```python
from build123d import *

# Parameters (mm, degrees)
IZIM1_W                     = 100
IZIM1_H                     = 120
Y_KSEKLIK_EKSTR_ZYON1_DEPTH = 20
Y_KSEKLIK_EKSTR_ZYON2_DEPTH = 120
Y_KSEKLIK_EKSTR_ZYON3_DEPTH = 20
RADYUS1_R                   = 10
RADYUS2_R                   = 15
IZIM3_R                     = 20
Y_KSEKLIK_EKSTR_ZYON4_DEPTH = 30
IZIM4_R                     = 5
Y_KSEKLIK_EKSTR_ZYON5_DEPTH = 10
Y_KSEKLIK_EKSTR_ZYON6_START = 30
IZIM5_R                     = 20
Y_KSEKLIK_EKSTR_ZYON6_DEPTH = 30
Y_KSEKLIK_EKSTR_ZYON7_START = 10
IZIM6_R                     = 5
Y_KSEKLIK_EKSTR_ZYON7_DEPTH = 10


with BuildPart() as part:
    # Çizim1 → Yükseklik-Ekstrüzyon1 (new body)
    with BuildSketch(Plane.XY):
        Rectangle(IZIM1_W, IZIM1_H)
    extrude(amount=Y_KSEKLIK_EKSTR_ZYON1_DEPTH)

    # Çizim1<3> → Yükseklik-Ekstrüzyon2 (add)
    with BuildSketch(Plane.XY):
        with BuildLine():
            Line((-50, -60), (-50, 60))
            ThreePointArc((-50, 60), (-110, 0), (-50, -60))
        make_face()
    extrude(amount=Y_KSEKLIK_EKSTR_ZYON2_DEPTH)

    # Çizim2 → Yükseklik-Ekstrüzyon3 (add)
    with BuildSketch(Plane.XY.offset(120)):
        with BuildLine():
            Line((-50, -60), (50, -60))
            Line((50, -60), (50, 60))
            Line((50, 60), (-50, 60))
            ThreePointArc((-50, 60), (-110, 0), (-50, -60))
        make_face()
    extrude(amount=Y_KSEKLIK_EKSTR_ZYON3_DEPTH)

    # Radyus1
    radyus1_edges = [part.edges().sort_by_distance(p)[0] for p in [
        (-50, 0, 120),
        (-50, 0, 20),
    ]]
    fillet(radyus1_edges, radius=RADYUS1_R)

    # Radyus2
    radyus2_edges = [part.edges().sort_by_distance(p)[0] for p in [
        (50, -60, 130),
        (50, 60, 130),
        (50, 60, 10),
        (50, -60, 10),
    ]]
    fillet(radyus2_edges, radius=RADYUS2_R)

    # Çizim3 → Yükseklik-Ekstrüzyon4 (add)
    with BuildSketch(Plane.XY.offset(20)):
        Circle(IZIM3_R)
    extrude(amount=Y_KSEKLIK_EKSTR_ZYON4_DEPTH)

    # Çizim4 → Yükseklik-Ekstrüzyon5 (add)
    with BuildSketch(Plane.XY.offset(50)):
        Circle(IZIM4_R)
    extrude(amount=Y_KSEKLIK_EKSTR_ZYON5_DEPTH)

    # Çizim5 → Yükseklik-Ekstrüzyon6 (add)
    with BuildSketch(Plane(origin=(0, 0, 120), x_dir=(1, 0, 0), z_dir=(0, 0, -1)).offset(Y_KSEKLIK_EKSTR_ZYON6_START)):
        Circle(IZIM5_R)
    extrude(amount=-Y_KSEKLIK_EKSTR_ZYON6_DEPTH)

    # Çizim6 → Yükseklik-Ekstrüzyon7 (add)
    with BuildSketch(Plane(origin=(0, 0, 90), x_dir=(1, 0, 0), z_dir=(0, 0, -1)).offset(Y_KSEKLIK_EKSTR_ZYON7_START)):
        Circle(IZIM6_R)
    extrude(amount=-Y_KSEKLIK_EKSTR_ZYON7_DEPTH)


solid = part.part
```
Check sheet for the modelled part. Datum: model origin and axes. Units: mm. A direction names the side the tool comes from. Coordinates: 2 decimals unless noted, no trailing zeros. Write each loop counter-clockwise with the first axis right and the second up, starting at its lowest first coordinate (ties: lowest second). Pieces come first, ordered by that corner, then holes. Notation, with made-up numbers: (11, 43) -> (62, 43) arc R16 cw to (62, 54) -> close; hole circle Ø9 at (47, 44.25). An arc over 180 degrees is marked (long way). Use a Markdown table: item, result.
1. Scan lines: line 1 along Z through (x, y) = (-18.5, 17); line 2 along X through (y, z) = (0.5, 59.5); line 3 along Z through (x, y) = (-12, 4). Record each from-to range of solid material in increasing order.
Reported:
| item | result |
|---|---|
| line 1 | z = 0 to 20, 120 to 140 |
| line 2 | x = -110 to -50, -4.97 to 4.97 |
| line 3 | z = 0 to 50, 90 to 140 |
2. Tool access check on faces 3 (the cylindrical face through (45.72, -55.49, 10.14)), 4 (the flat face through (4, 4, 90)), 5 (the flat face through (-50, -1, 69)), 6 (the flat face through (50, -1, 10)), 7 (the flat face through (0, 0, 60)). Record the directions out of +Z, -Z, +X, -X, +Y, -Y that give a thin tool (end or side, any length) a straight path to the whole face; none if there is none.
Reported:
| item | result |
|---|---|
| face 3 | +Z, -Z, +X, -Y |
| face 4 | none |
| face 5 | +Y, -Y |
| face 6 | +Z, -Z, +X, +Y, -Y |
| face 7 | +X, +Y, -Y |
3. Go/stop test with flat-tipped pins: pin 1 Ø10 at (x, z) = (-13, 78) entering from -Y; pin 2 Ø5 at (y, z) = (36, 23) entering from -X; pin 3 Ø8 at (y, z) = (32.5, 87) entering from +X. Record where each tip stops, or that it passes through.
Reported:
| item | result |
|---|---|
| pin 1 | passes through |
| pin 2 | stops at x = -99.78 |
| pin 3 | stops at x = -50 |
4. Sectioned sample at A-A (x = 0). Enter the section's corners in (y, z).
Reported:
| item | result |
|---|---|
| outline | (-60, 0) -> (60, 0) -> (60, 20) -> (20, 20) -> (20, 50) -> (5, 50) -> (5, 60) -> (-5, 60) -> (-5, 50) -> (-20, 50) -> (-20, 20) -> (-60, 20) -> close; (-60, 120) -> (-20, 120) -> (-20, 90) -> (-5, 90) -> (-5, 80) -> (5, 80) -> (5, 90) -> (20, 90) -> (20, 120) -> (60, 120) -> (60, 140) -> (-60, 140) -> close |
5. Sectioned sample at C-C (y = 36). Enter the section's corners in (x, z), plus the area to 3 significant figures.
Reported:
| item | result |
|---|---|
| outline | (-98, 0) -> (50, 0) -> (50, 20) -> (-40, 20) arc R10 cw to (-50, 30) -> (-50, 110) arc R10 cw to (-40, 120) -> (50, 120) -> (50, 140) -> (-98, 140) -> close |
| area | 10,800 mm2 |
6. Sectioned sample at D-D (z = 35.5). Enter the section's corners in (x, y).
Reported:
| item | result |
|---|---|
| outline | (-50, -60) -> (-50, 60) arc R60 ccw to start; circle Ø40 at (0, 0) |
7. Release check for a two-part mould opening along Z. For faces 1 (the cylindrical face through (45.49, -55.72, 130.14)), 2 (the cylindrical face through (-46.99, 0.84, 117.15)) record: pulls with the +Z half, pulls with the -Z half, needs draft (parallel to the pull), parting line crosses it, or undercut.
Reported:
| item | result |
|---|---|
| face 1 | needs draft |
| face 2 | undercut |
8. Sectioned sample at B-B (z = 14). Enter the section's corners in (x, y), plus the area to 3 significant figures.
Reported:
| item | result |
|---|---|
| outline | (-50, -60) -> (35, -60) arc R15 ccw to (50, -45) -> (50, 45) arc R15 ccw to (35, 60) -> (-50, 60) arc R60 ccw to start |
| area | 17,600 mm2 |
